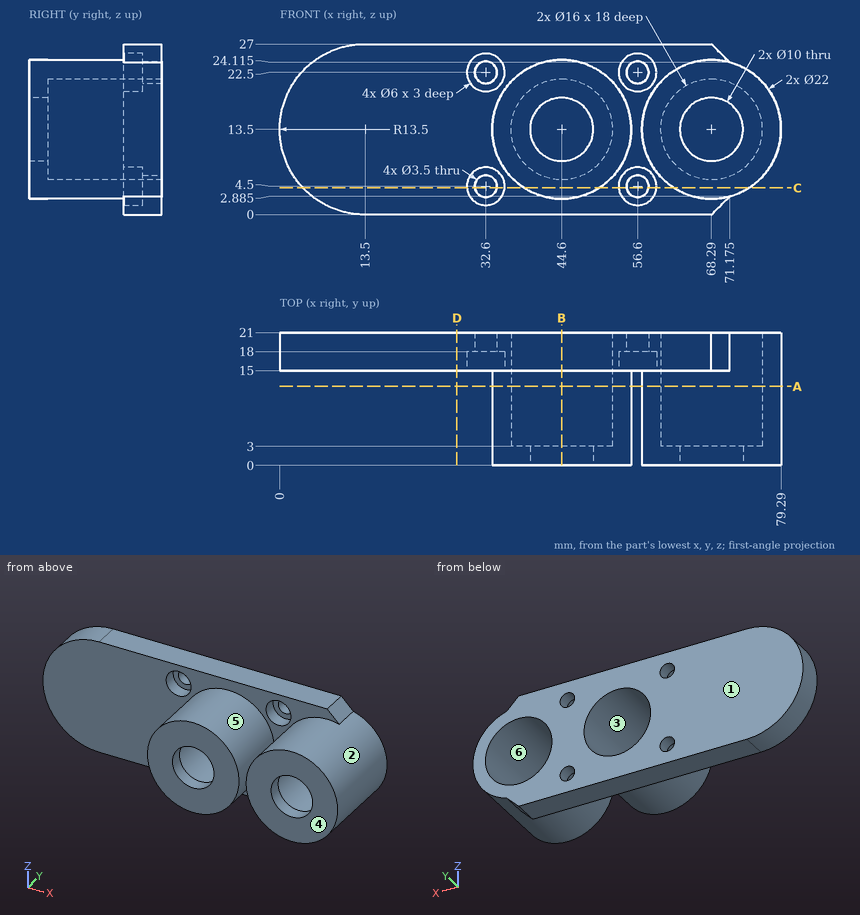
Could you check a few things on this drawing? It's one solid part, dimensions in mm from its lowest x, y, z. A direction names the side the tool comes from. Give positions to 0.01 mm unless a question says otherwise; leave off trailing zeros. Write each loop counter-clockwise with the first axis right and the second up, starting at its lowest first coordinate (ties: lowest second). Pieces come first, ordered by that corner, then holes. Notation, with made-up numbers: (-27.75, 12.5) - (28.25, 12.5) arc R20 ccw to (28.25, 38.5) - close; hole circle Ø2 at (65, 44). An arc over 180 degrees is marked (long way). Use CSV: the item, a comma, the result in double quotes. Start each with the question number.
Item 1: If I drill on line 1 along Z through (x, y) = (32.6, 20.1); line 2 along X through (y, z) = (16.55, 4.5) (1 decimal); line 3 along Y through (x, z) = (38.5, 16.75), over which ranges is the centre line in solid material (lowest first)?
Item 2: If we mould it in two halves opening along Z, with no side actions, what happens to the marked faces 4, 5 and 6? For each: pulls with the +Z half, pulls with the -Z half, needs draft (parallel to the pull), parting line crosses it, or undercut.
Item 3: I want a section at B-B, the plane x = 44.6. Please give me the cut outline in (y, z).
Item 4: I want a section at C-C, the plane z = 4.25. Please give me the cut outline in (x, y).
Item 5: For the marked faces 1, 2 and 3, which set-ups out of +Z, -Z, +X, -X, +Y, -Y let a thin tool reach every point of the face, with its end or its side?
Item 6: I want a section at D-D, the plane x = 28. Please give me the cut outline in (y, z), then the cut area to 3 significant figures.
Item 7: I want a section at A-A, the plane y = 12.5. Please give me the cut outline in (x, z), then the cut area to 3 significant figures.
Item 8: I'm going to push flat-ended pins straight in: pin 1 (10 mm diameter, centred on x = 42, z = 21, fed in from +Y); pin 2 (3 mm diameter, centred on x = 32, z = 21.5, fed in from -Y); pin 3 (3 mm diameter, centred on x = 11, z = 3.5, fed in from -Y); pin 4 (4 mm diameter, centred on y = 7, z = 22.5, fed in from +X) (1 decimal). Where does each tip first touch, or does it pass through?
Findings:
1,line 1,"z = 0 to 2.75, 6.25 to 20.75, 24.25 to 27"
1,line 2,"x = 3.4 to 29.6, 35.6 to 53.6, 59.6 to 74.6"
1,line 3,"y = 0 to 3"
2,face 4,"needs draft"
2,face 5,"parting line crosses it"
2,face 6,"undercut"
3,outline,"(0, 2.5) - (15, 2.5) - (15, 0) - (21, 0) - (21, 5.5) - (3, 5.5) - (3, 8.5) - (0, 8.5) - close; (0, 18.5) - (3, 18.5) - (3, 21.5) - (21, 21.5) - (21, 27) - (15, 27) - (15, 24.5) - (0, 24.5) - close"
4,outline,"(3.67, 15) - (29.61, 15) - (29.61, 18) - (30.87, 18) - (30.87, 21) - (3.67, 21) - close; (34.33, 18) - (35.59, 18) - (35.59, 15) - (38.65, 15) - (38.65, 0) - (50.55, 0) - (50.55, 15) - (53.61, 15) - (53.61, 18) - (54.87, 18) - (54.87, 21) - (34.33, 21) - close; (58.33, 18) - (59.59, 18) - (59.59, 15) - (62.34, 15) - (62.34, 0) - (74.24, 0) - (74.24, 21) - (58.33, 21) - close"
5,face 1,"+Z, -Z, +X, -X, +Y"
5,face 2,"-Y"
5,face 3,"+Y"
6,outline,"(15, 0) - (21, 0) - (21, 27) - (15, 27) - close"
6,area,"162 mm2"
7,outline,"circle Ø22 at (44.6, 13.5); circle Ø22 at (68.29, 13.5); hole circle Ø16 at (44.6, 13.5); hole circle Ø16 at (68.29, 13.5)"
7,area,"358 mm2"
8,pin 1,"stops at y = 21"
8,pin 2,"stops at y = 18"
8,pin 3,"stops at y = 15"
8,pin 4,"stops at x = 76.8"
